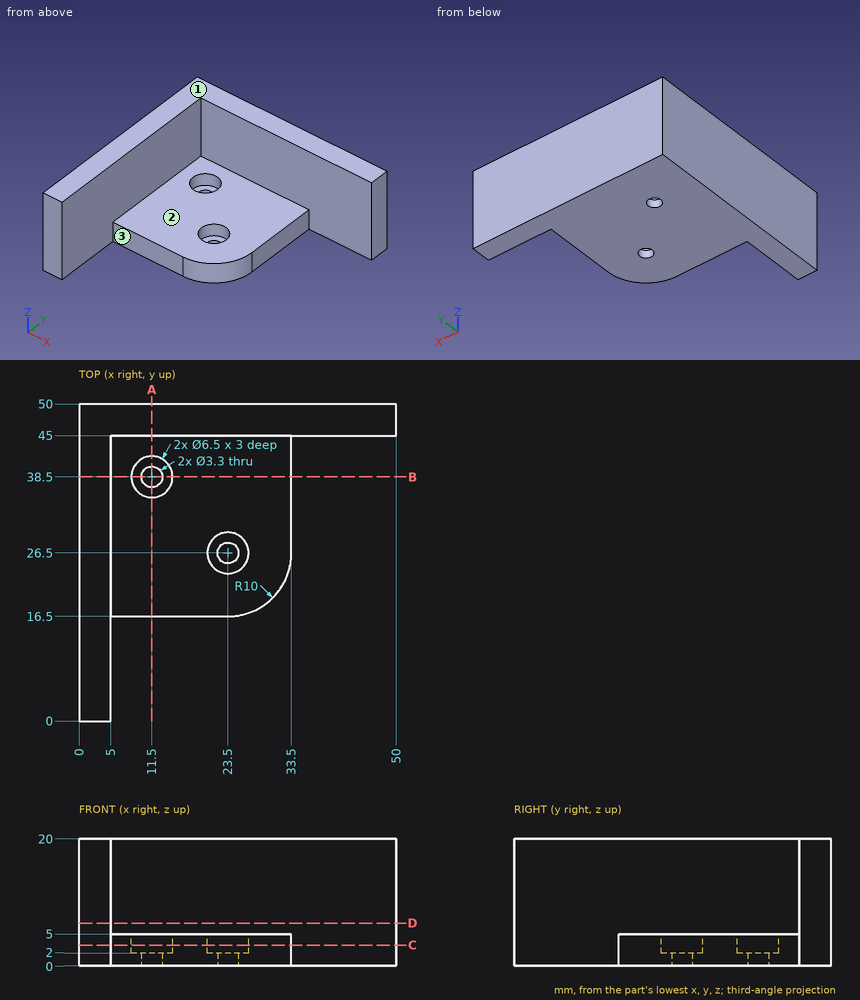
For this review, use the dimensioned drawing (mm, ordinates from the lowest corner) and the shaded views. A direction names the side the tool comes from. Coordinates: 2 decimals unless noted, no trailing zeros. Write each loop counter-clockwise with the first axis right and the second up, starting at its lowest first coordinate (ties: lowest second). Pieces come first, ordered by that corner, then holes. Notation, with made-up numbers: (5.5, -24.75) - (53.5, -24.75) arc R18 ccw to (53.5, 8.25) - close; hole circle Ø8 at (24.5, 65.25). An arc over 180 degrees is marked (long way). Answer as a JSON object with one key per item and string values. Group by question number.
1. Add section D-D (z = 6.75). Give the boundary of the cut face in (x, y).
2. Add section A-A (x = 11.5). Give the boundary of the cut face in (y, z), plus the area to 3 significant figures.
3. Add section C-C (z = 3.25). Give the boundary of the cut face in (x, y), plus the area to 3 significant figures.
4. Machinability: for the marked faces 1, 2 and 3, which of the approach directions +Z, -Z, +X, -X, +Y, -Y give a long, thin tool a straight path to every point of the face, cutting with its end or side? Answer none if there is none.
5. Add section B-B (y = 38.5). Give the boundary of the cut face in (x, z).
6. To check wall thickness, follow probe 1 along Y at (x, z) = (11.5, 0.5); probe 2 along X at (y, z) = (26.5, 3.3); probe 3 along Y at (x, z) = (11.5, 2.9). State the ranges of each line that lie inside material, in increasing order.
7. Clearance check with flat-ended pins moving along their axes: pin 1 Ø8 at (y, z) = (40, 12.5) entering from +X; pin 2 Ø7 at (x, y) = (23, 25.5) entering from +Z; pin 3 Ø6 at (x, z) = (25.5, 7) entering from -Y. State where each tip first meets the part, or that it passes through.
Findings:
{
 "1": {"outline": "(0, 0) - (5, 0) - (5, 45) - (50, 45) - (50, 50) - (0, 50) - close"},
 "2": {"outline": "(16.5, 0) - (36.85, 0) - (36.85, 2) - (35.25, 2) - (35.25, 5) - (16.5, 5) - close; (40.15, 0) - (50, 0) - (50, 20) - (45, 20) - (45, 5) - (41.75, 5) - (41.75, 2) - (40.15, 2) - close", "area": "216 mm²"},
 "3": {"outline": "(0, 0) - (5, 0) - (5, 16.5) - (23.5, 16.5) arc R10 ccw to (33.5, 26.5) - (33.5, 45) - (50, 45) - (50, 50) - (0, 50) - close; hole circle Ø6.5 at (11.5, 38.5); hole circle Ø6.5 at (23.5, 26.5)", "area": "1,200 mm²"},
 "4": {"face 1": "+Z, +X, -X, +Y, -Y", "face 2": "+Z, +X, -Y", "face 3": "+Z, -Z, +X, -Y"},
 "5": {"outline": "(0, 0) - (9.85, 0) - (9.85, 2) - (8.25, 2) - (8.25, 5) - (5, 5) - (5, 20) - (0, 20) - close; (13.15, 0) - (33.5, 0) - (33.5, 5) - (14.75, 5) - (14.75, 2) - (13.15, 2) - close"},
 "6": {"probe 1": "16.5 to 36.85, 40.15 to 50", "probe 2": "0 to 20.25, 26.75 to 33.5", "probe 3": "16.5 to 35.25, 41.75 to 50"},
 "7": {"pin 1": "x = 5", "pin 2": "z = 5", "pin 3": "y = 16.5"}
}
